from build123d import *


# Not quite as in the source:
# - a feature names something its author has since deleted; it is built from what else it names


with BuildPart() as f1:
    # F0 (on Right) → F1 (revolve)
    with BuildSketch(Plane.YZ):
        with BuildLine():
            Line((21.5, 4), (21.5, 0))
            Line((21.5, 0), (24.5, 0))
            Line((24.5, 0), (24.5, 1.7079167301))
            Line((24.5, 1.7079167301), (24.5, 12.5))
            ThreePointArc((24.5, 12.5), (24.2071067812, 13.2071067812), (23.5, 13.5))
            Line((23.5, 13.5), (0, 13.5))
            Line((0, 13.5), (0, 12.5))
            Line((0, 12.5), (22.5, 12.5))
            Line((22.5, 12.5), (23.5, 12.5))
            Line((23.5, 12.5), (23.5, 7.5))
            Line((23.5, 7.5), (22.5, 7.5))
            Line((22.5, 7.5), (22.5, 4))
            Line((22.5, 4), (21.5, 4))
        make_face()
        with BuildLine():
            Line((24.5, 1.7079167301), (24.5, 0))
            ThreePointArc((24.5, 0), (25.353958365, 0.853958365), (24.5, 1.7079167301))
        make_face()
    revolve(axis=Axis((0, 0, 6.75), (0, 0, 1)))


solid = f1.part
Read the model definition and answer for the solid it produces. Units are mm, in the model's axes. A direction names the side the tool comes from. Give positions to 0.01 mm unless a question says otherwise; leave off trailing zeros. Loops run counter-clockwise (first coordinate to the right, second up) from the corner with the lowest first, then second, coordinate; pieces in that order, holes last. Notation, with made-up numbers: (-14.75, 36.5) - (12.25, 36.5) arc R22 cw to (12.25, 47.5) - close; hole circle Ø7 at (-19.75, 31). An arc over 180 degrees is marked (long way). Answer as CSV lines item,"result". Start each with the question number.
1) Find section A-A (x = 0). Write down the section's boundary in (y, z).
2) Find section B-B (z = 11). Write down the section's boundary in (x, y), then the cut area to 3 significant figures.
3) Determine the mould class of faces 1 (the face through (-20.66, 13.17, 7.18)), 2 (the face through (0, 0, 13.5)), 3 (the face through (-7.1, 22.4, 10)), 4 (the face through (0, 23, 7.5)) for opening direction X: released by +X, released by -X, zero draft, split by the parting line, or undercut.
4) Find section D-D (z = 6). Write down the section's boundary in (x, y).
5) Straight lines are drawn through the part: L1, parallel to Y at x = 0, z = 5.85; L2, parallel to Y at x = 0, z = 9.75; L3, parallel to Z at x = 19, y = -13. For each, find the intervals that lie inside material, in ascending order. Write a range as from..to.
6) Which of the six approach directions +Z, -Z, +X, -X, +Y, -Y give full straight-line access (tool end or side, diameter ignored) to faces 5 (the face through (2, 22, 4)), 6 (the face through (-21.317, -2.799, 1.972)), 7 (the face through (22, 0, 0))?
7) Each of these flat-tipped pins is pushed along its axis until it touches: pin 1 Ø6 at (y, z) = (10, 4) entering from -X (3 decimals); pin 2 Ø14 at (x, y) = (-1, -7) entering from -Z; pin 3 Ø1.5 at (x, z) = (16, 11) entering from -Y. Where does it stop, or does it pass through?
Findings below:
1,outline,"(-24.5, 0) - (-21.5, 0) - (-21.5, 4) - (-22.5, 4) - (-22.5, 7.5) - (-23.5, 7.5) - (-23.5, 12.5) - (23.5, 12.5) - (23.5, 7.5) - (22.5, 7.5) - (22.5, 4) - (21.5, 4) - (21.5, 0) - (24.5, 0) arc R0.85 ccw to (24.5, 1.71) - (24.5, 12.5) arc R1 ccw to (23.5, 13.5) - (-23.5, 13.5) arc R1 ccw to (-24.5, 12.5) - (-24.5, 1.71) arc R0.85 ccw to start"
2,outline,"circle Ø49 at (0, 0); hole circle Ø47 at (0, 0)"
2,area,"151 mm^2"
3,face 1,"split by the parting line"
3,face 2,"zero draft"
3,face 3,"undercut"
3,face 4,"undercut"
4,outline,"circle Ø49 at (0, 0); hole circle Ø45 at (0, 0)"
5,L1,"-24.5..-22.5, 22.5..24.5"
5,L2,"-24.5..-23.5, 23.5..24.5"
5,L3,"0..7.5, 12.5..13.5"
6,face 5,"none"
6,face 6,"-Z"
6,face 7,"-Z, +X, -X, +Y, -Y"
7,pin 1,"x = -23.685"
7,pin 2,"z = 12.5"
7,pin 3,"y = -19.18"
